The model under review builds one solid part; all positions refer to its coordinate system, in mm. Face numbers are marked on the shaded views. A direction names the side the tool comes from. Round coordinates to 2 decimals unless told otherwise and drop trailing zeros. Order: outer loops, then holes, each group sorted by start corner. A loop starts at its lowest first (then second) coordinate and runs counter-clockwise, first axis right, second up.
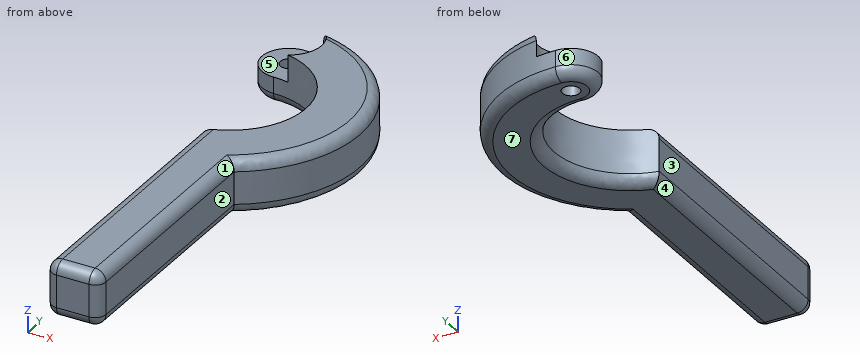
from build123d import *

# Parameters (mm, degrees)
F2_W     = 10
F2_H     = 10
F4_R     = 5
F5_DEPTH = 5
F6_R     = 6
F7_DEPTH = 5.0010001
F8_R     = 1.6
F9_DEPTH = 10.0010001
F10_R    = 2


with BuildPart() as f3:
    # F3: sweep along a path in F0
    with BuildLine(Plane.XY) as f3_path:
        ThreePointArc((0, 14), (13.943630847, 1.2550533066), (2.5, -13.774977314))
        Line((2.5, -13.774977314), (2.5, -63.774977314))
    # F2 (on plane+point) → F3 (sweep)
    with BuildSketch(Plane.XZ.offset(63.774977314)):
        with Locations((7.5, 5)):
            Rectangle(F2_W, F2_H)
    sweep(path=f3_path.line, transition=Transition.RIGHT)

    # F4 (on Top) → F5 (join)
    with BuildSketch(Plane.XY):
        with Locations((0, 19)):
            Circle(F4_R)
    extrude(amount=F5_DEPTH)

    # F6 (on face) → F7 (cut, through all)
    with BuildSketch(Plane.XY.offset(5)):
        with Locations((0, 19)):
            Circle(F6_R)
    extrude(amount=F7_DEPTH, mode=Mode.SUBTRACT)

    # F8 (on Top) → F9 (cut, through all)
    with BuildSketch(Plane.XY):
        with Locations((0, 19)):
            Circle(F8_R)
    extrude(amount=F9_DEPTH, mode=Mode.SUBTRACT)

    # F10
    f10_edges = [f3.edges().sort_by_distance(p)[0] for p in [
        (2.5, -38.774977, 10),
        (2.5, -38.774977, 0),
        (2.5, -63.774977, 5),
        (12.5, -63.774977, 5),
        (12.5, -42.131389, 10),
        (23.539652, 4.67812, 10),
        (12.5, -42.131389, 0),
        (7.5, -63.774977, 0),
        (7.5, -63.774977, 10),
        (13.943631, 1.255053, 0),
    ]]
    fillet(f10_edges, radius=F10_R)


solid = f3.part
(1) Clearance check with flat-ended pins moving along their axes: P1, Ø12, axis at x = 8.5, y = -5.5, coming from the -Z side; P2, Ø2, axis at y = -32.5, z = 3.5, coming from the +X side; P3, Ø3, axis at y = -9.5, z = 6.5, coming from the +X side; P4, Ø4, axis at x = 3, z = 5.5, coming from the +Y side. State where each tip first meets the part, or that it passes through.
(2) Tool access review of the marked faces 1, 2, 3 and 4: name each direction out of +Z, -Z, +X, -X, +Y, -Y from which nothing blocks a thin tool from reaching the whole face with its end or side.
(3) We need section A-A (y = -25.5). Give the boundary of the cut face in (x, z), and give its area (3 significant figures).
(4) To check wall thickness, follow L1, parallel to Y at x = 4, z = 5.5; L2, parallel to X at y = -42.5, z = 3.5; L3, parallel to X at y = 19, z = 3.35. State the ranges of each line that lie inside material, in increasing order.
(5) The part is to be moulded in two halves that separate along Y. For the marked faces 5, 6 and 7, say which applies: pulls with the +Y half, pulls with the -Y half, needs draft (parallel to the pull), parting line crosses it, or undercut.
Verdict:
1. P1: stops at z = 0
1. P2: stops at x = 12.5
1. P3: stops at x = 22.63
1. P4: stops at y = 23.98
2. face 1: +Z, +X, -Y
2. face 2: +Z, -Z, +X, -Y
2. face 3: +Z, -Z, -X, -Y
2. face 4: -Z, -X, -Y
3. outline: (2.5, 2) arc R2 ccw to (4.5, 0) - (10.5, 0) arc R2 ccw to (12.5, 2) - (12.5, 8) arc R2 ccw to (10.5, 10) - (4.5, 10) arc R2 ccw to (2.5, 8) - close
3. area: 96.6 mm2
4. L1: y = -63.71 to -13.42, 13.42 to 14.53, 23.47 to 23.66
4. L2: x = 2.5 to 12.5
4. L3: x = -5 to -1.6, 1.6 to 14.66
5. face 5: undercut
5. face 6: parting line crosses it
5. face 7: needs draft
